Verification items for the finished model (mm, model axes). A direction names the side the tool comes from. Coordinates: 2 decimals unless noted, no trailing zeros. Order: outer loops, then holes, each group sorted by start corner. A loop starts at its lowest first (then second) coordinate and runs counter-clockwise, first axis right, second up. Notation, with made-up numbers: M -15.5,57.5 L 15.5,57.5 A35 ccw 15.5,90.5 Z; hole C 71,36.25 d7. An arc over 180 degrees is marked long. Return JSON: item names as keys, results as strings. Group by question number.
Q1. Access from +Z, -Z, +X, -X, +Y, -Y to the whole of each face (thin tool, end or side, straight path). Record for faces 1 (the face through (44, 5, 0)), 2 (the face through (49.3, 3, 1.3)), 3 (the face through (28, 4, 0)).
Q2. Go/stop test with flat-tipped pins: pin 1 Ø5 at (x, z) = (48, 0) entering from +Y; pin 2 Ø2 at (y, z) = (12.5, 4) entering from +X; pin 3 Ø2.5 at (x, z) = (38, 0) entering from -Y; pin 4 Ø7 at (x, z) = (-0.5, 0.5) entering from -Y. Record where each tip stops, or that it passes through.
Q3. Section check C-C, the plane x = 48. Enter the section's corners in (y, z).
Q4. Section check D-D, the plane x = 9.5. Enter the section's corners in (y, z).
Q5. Section check A-A, the plane x = 0. Enter the section's corners in (y, z), then the cut area to 3 significant figures.
Q6. Thickness scan on probe 1 along X at (y, z) = (3.8, 0); probe 2 along Z at (x, y) = (48, 4.35); probe 3 along X at (y, z) = (1.25, 0). Record the ranges inside material, lowest first.
Q7. Mould release check, pull along X, two halves, no side actions. Record for faces 4 (the face through (3.3, 7, 0.1)), 5 (the face through (1.43, 7.99, -2.75)), 6 (the face through (-6, 14, 0)), 7 (the face through (34.926, 3.986, -0.404)): pulls with the +X half, pulls with the -X half, needs draft (parallel to the pull), parting line crosses it, or undercut.
Q8. Section check B-B, the plane z = 0. Count the separate pieces of the cut face and the enclosed holes in it, then the cut area to 3 significant figures.
Autodesk Inventor part; units mm, degrees
ref_plane "YZ Plane" through (0, 0, 0) normal (1, 0, 0) x (0, 1, 0)
ref_plane "XZ Plane" through (0, 0, 0) normal (0, 1, 0) x (-1, 0, 0)
ref_plane "XY Plane" through (0, 0, 0) normal (0, 0, 1) x (1, 0, 0)
sketch "Sketch1" plane through (0, 0, 0) normal (0, 0, 1) x (1, 0, 0)
  line L0 (0, 0) -> (0, 15)
  line L1 (0, 15) -> (23.6569, 15)
  line L2 (21, 12) -> (0, 12)
  line L3 (0, 12) -> (0, 15)
  line L4 (28, 0) -> (55, 0)
  line L5 (55, 0) -> (55, 5)
  line L6 (55, 5) -> (28, 5)
  line L7 (28, 5) -> (28, 0)
  line L8 (28, 5) -> (21, 12)
  line L9 (23.6569, 15) -> (33.6569, 5)
  dimension "d0" = 135
  dimension "d1" = 5
  dimension "d2" = 28
  dimension "d3" = 3
  dimension "d4" = 4
  dimension "d5" = 12
  dimension "d6" = 55
extrude "Extrusion1" add sketch "Sketch1" along normal mid plane 10
sketch "Sketch3" plane through (33.6569, 5, 5) normal (0, 1, 0) x (1, 0, 0)
  line L0 (21.3431, 10) -> (21.3431, 0)
  line L1 (21.3431, 5) -> (-0.1629, 5) construction
  line L2 (-33.6569, 0) -> (-33.6569, 10)
  point P0 (-33.6569, 5)
  point P1 (14.3431, 5)
  point P2 (4.3431, 5)
  dimension "d9" = 10
  dimension "d18" = 38
hole "Hole1" at (48, 5, 0) at (38, 5, 0) direction (0, -1, 0) diameter 3.2 end through all counterbore diameter 6.2 counterbore depth 2
chamfer "Chamfer1" distance 2 angle 45 1 edges at (28, 0, 0)
sketch "Sketch4" plane through (0, 15, 5) normal (0, 1, 0) x (1, 0, 0)
  circle A0 centre (0, 5) radius 6
  dimension "d22" = 12
extrude "Extrusion2" add sketch "Sketch4" against normal up to surface (3 mm away)
sketch "Sketch5" plane through (21, 12, -5) normal (0, -1, 0) x (1, 0, 0)
  circle A0 centre (-21, 5) radius 6
  arc A1 (-17.6834, 10) -> (-17.6834, 0) centre (-21, 5) ccw
extrude "Extrusion3" add sketch "Sketch5" along normal blind 1
sketch "Sketch6" plane through (0, 11, 0) normal (0, -1, 0) x (1, 0, 0)
  circle A0 centre (0, 0) radius 5
  point P0 (0, 0)
  dimension "d27" = 10
extrude "Extrusion4" add sketch "Sketch6" along normal blind 4
sketch "Sketch7" plane through (0, 7, 0) normal (0, -1, 0) x (1, 0, 0)
  circle A0 centre (0, 0) radius 3.1
  point P0 (0, 0)
  dimension "d30" = 6.2
extrude "Extrusion5" cut sketch "Sketch7" against normal blind 2
sketch "Sketch8" plane through (23.6569, 15, 5) normal (0, 1, 0) x (1, 0, 0)
  circle A0 centre (-23.6569, 5) radius 1.6
  dimension "d33" = 3.2
extrude "Extrusion6" cut sketch "Sketch8" against normal through all
chamfer "Chamfer2" [suppressed]
fillet "Fillet1" radius 2 2 edges at (55, 2.5, 5) (55, 2.5, -5)
properties part number "joint mag"
Numbers:
{
 "1": {"face 1": "+Z, -Z, +X, +Y", "face 2": "+Y", "face 3": "+Z, -Z, -X, -Y"},
 "2": {"pin 1": "stops at y = 3", "pin 2": "stops at x = 27.16", "pin 3": "passes through", "pin 4": "stops at y = 7"},
 "3": {"outline": "M 0,-5 L 5,-5 L 5,-3.1 L 3,-3.1 L 3,-1.6 L 0,-1.6 Z; M 0,1.6 L 3,1.6 L 3,3.1 L 5,3.1 L 5,5 L 0,5 Z"},
 "4": {"outline": "M 12,-5 L 15,-5 L 15,5 L 12,5 Z"},
 "5": {"outline": "M 7,-5 L 11,-5 L 11,-6 L 15,-6 L 15,-1.6 L 9,-1.6 L 9,-3.1 L 7,-3.1 Z; M 7,3.1 L 9,3.1 L 9,1.6 L 15,1.6 L 15,6 L 11,6 L 11,5 L 7,5 Z", "area": "56.4 mm2"},
 "6": {"probe 1": "x = 28 to 34.9, 41.1 to 44.9, 51.1 to 55", "probe 2": "z = -5 to -3.1, 3.1 to 5", "probe 3": "x = 28.75 to 36.4, 39.6 to 46.4, 49.6 to 55"},
 "7": {"face 4": "needs draft", "face 5": "undercut", "face 6": "parting line crosses it", "face 7": "undercut"},
 "8": {"separate pieces": "4", "enclosed holes": "0", "area": "242 mm2"}
}
